```python
from build123d import *

# Parameters (mm, degrees)
SKETCH1_W                   = 210.475
SKETCH1_H                   = 9.525
BOSS_EXTRUDE1_DEPTH         = 63.9
SKETCH2_W                   = 40
SKETCH2_H                   = 20
CUT_EXTRUDE1_DEPTH          = 10.525
FILLET1_R                   = 12.7
TAP_DRILL_FOR_M4_TAP1_D     = 3.3
TAP_DRILL_FOR_M4_TAP1_DEPTH = 12.7
TAP_DRILL_FOR_M4_TAP1_TIP   = 0.991420021
CUT_EXTRUDE2_DEPTH          = 10.525


with BuildPart() as part:
    # Sketch1 → Boss-Extrude1 (new body)
    with BuildSketch(Plane.XY):
        Rectangle(SKETCH1_W, SKETCH1_H)
    extrude(amount=BOSS_EXTRUDE1_DEPTH)

    # Sketch2 → Cut-Extrude1 (cut, through all)
    with BuildSketch(Plane(origin=(0, 4.7625, 0), x_dir=(1, 0, 0), z_dir=(0, 1, 0))):
        with Locations((-19.7625, -10)):
            Rectangle(SKETCH2_W, SKETCH2_H)
    extrude(amount=-CUT_EXTRUDE1_DEPTH, mode=Mode.SUBTRACT)

    # Fillet1
    fillet1_edges = [part.edges().sort_by_distance(p)[0] for p in [
        (-39.7625, 0, 20),
        (0.2375, 0, 20),
    ]]
    fillet(fillet1_edges, radius=FILLET1_R)

    # Tap Drill for M4 Tap1
    with Locations(Plane.XY.offset(63.9)):
        with Locations((-76.2285, 0), (2.6995, 0), (81.6285, 0)):
            Hole(TAP_DRILL_FOR_M4_TAP1_D / 2, depth=TAP_DRILL_FOR_M4_TAP1_DEPTH)
            with Locations((0, 0, -(TAP_DRILL_FOR_M4_TAP1_DEPTH + TAP_DRILL_FOR_M4_TAP1_TIP / 2))):  # 118° drill point
                Cone(0, TAP_DRILL_FOR_M4_TAP1_D / 2, TAP_DRILL_FOR_M4_TAP1_TIP, mode=Mode.SUBTRACT)

    # Sketch7 → Cut-Extrude2 (cut, through all)
    with BuildSketch(Plane(origin=(0, 4.7625, 0), x_dir=(1, 0, 0), z_dir=(0, 1, 0))):
        with BuildLine():
            Line((43.2375, -37.9), (105.2375, -37.9))
            Line((105.2375, -37.9), (105.2375, -55.9))
            Line((105.2375, -55.9), (43.2375, -55.9))
            ThreePointArc((43.2375, -55.9), (34.2375, -46.9), (43.2375, -37.9))
        make_face()
    extrude(amount=-CUT_EXTRUDE2_DEPTH, mode=Mode.SUBTRACT)


solid = part.part
```
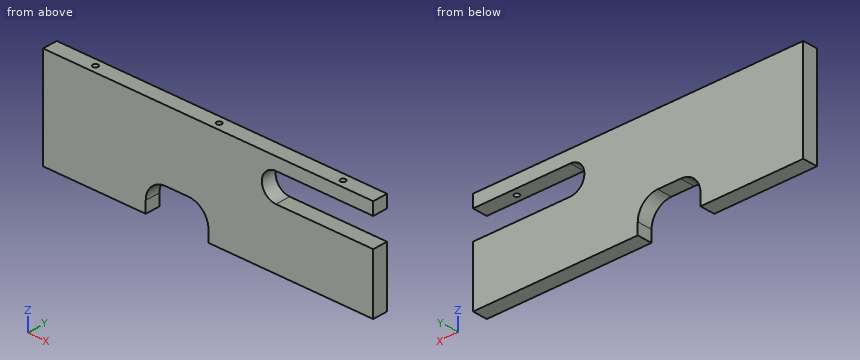
Check sheet for the modelled part. Datum: model origin and axes. Units: mm. Coordinates: 2 decimals unless noted, no trailing zeros. Write each loop counter-clockwise with the first axis right and the second up, starting at its lowest first coordinate (ties: lowest second). Pieces come first, ordered by that corner, then holes. Notation, with made-up numbers: M 31.5,43.25 L 72.5,43.25 A25 ccw 72.5,59.25 Z; hole C -20.5,10.5 d4. An arc over 180 degrees is marked long. Use one line per item in the form item = value.
Item 1: Sectioned sample at B-B, the plane z = 46.9. Record the cut outline in (x, y), and give its area (3 significant figures).
Answer below:
outline = M -105.24,-4.76 L 34.24,-4.76 L 34.24,4.76 L -105.24,4.76 Z
area = 1,330 mm^2
Item 2: Sectioned sample at A-A, the plane x = 38.5. Record the cut outline in (y, z).
Answer below:
outline = M -4.76,0 L 4.76,0 L 4.76,39.25 L -4.76,39.25 Z; M -4.76,54.55 L 4.76,54.55 L 4.76,63.9 L -4.76,63.9 Z
Item 3: Material ranges on L1, parallel to Z at x = 72.5, y = 0.5; L2, parallel to X at y = 0, z = 54.25; L3, parallel to X at y = 0, z = 54, recorded low to high. Write a range as from..to.
Answer below:
L1 = 0..37.9, 55.9..63.9
L2 = -105.24..-77.88, -74.58..1.05, 4.35..38.04
L3 = -105.24..-77.88, -74.58..1.05, 4.35..37.71
Item 4: Gauge pin test, flat ends, axial feed: pin 1 Ø3 at (x, y) = (2.7, 0) entering from +Z; pin 2 Ø2 at (x, y) = (-76.23, 0) entering from +Z; pin 3 Ø1.5 at (y, z) = (2.5, 49) entering from +X. Record the tip position at first contact, or that the pin passes through.
Answer below:
pin_1 = 51.11
pin_2 = 50.81
pin_3 = 34.7
